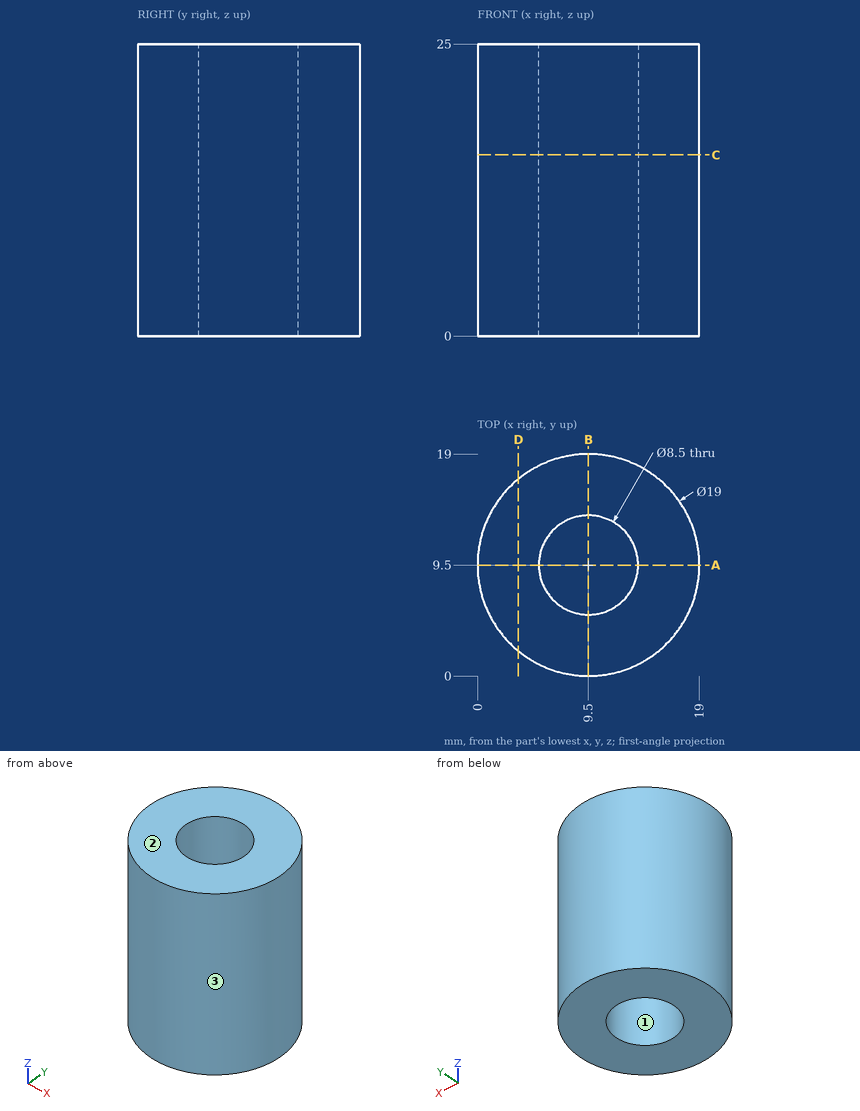
Job drawing, mm, ordinate dimensions from the low corner. One solid piece. Coordinates: 2 decimals unless noted, no trailing zeros. Write each loop counter-clockwise with the first axis right and the second up, starting at its lowest first coordinate (ties: lowest second). Pieces come first, ordered by that corner, then holes. Notation, with made-up numbers: M -17,44.25 L 22,44.25 A4 ccw 22,51.25 Z; hole C 60.25,79 d6. An arc over 180 degrees is marked long. Answer as a JSON object with one key per item and string values. Group by question number.
1) Pin check, flat tips, straight feed: pin 1 Ø1 at (x, z) = (13.5, 14.5) entering from +Y; pin 2 Ø5 at (x, z) = (5, 3) entering from -Y; pin 3 Ø1.5 at (y, z) = (16, 16.5) entering from -X. Stop position of each tip, or through.
2) Wall check: line 1 (Y direction, x = 9.5, z = 17); line 2 (Y direction, x = 7.5, z = 21.25); line 3 (X direction, y = 13, z = 14.75). Give the ranges that are in metal, low to high. Write a range as from..to.
3) Saw through at C-C (z = 15.5). Write the cut outline in (x, y).
4) Saw through at D-D (x = 3.5). Write the cut outline in (y, z).
5) Saw through at A-A (y = 9.5). Write the cut outline in (x, z), plus the area to 4 significant figures.
6) Mould opens along X. For the marked faces 1, 2 and 3 say: +X half, -X half, draft (parallel to the pull), parting line (faces both ways), or undercut.
Values follow:
{
 "1": {"pin 1": "stops at y = 18.33", "pin 2": "stops at y = 0.21", "pin 3": "stops at x = 1.94"},
 "2": {"line 1": "y = 0..5.25, 13.75..19", "line 2": "y = 0.21..5.75, 13.25..18.79", "line 3": "x = 0.67..7.09, 11.91..18.33"},
 "3": {"outline": "C 9.5,9.5 d19; hole C 9.5,9.5 d8.5"},
 "4": {"outline": "M 2.13,0 L 16.87,0 L 16.87,25 L 2.13,25 Z"},
 "5": {"outline": "M 0,0 L 5.25,0 L 5.25,25 L 0,25 Z; M 13.75,0 L 19,0 L 19,25 L 13.75,25 Z", "area": "262.5 mm2"},
 "6": {"face 1": "undercut", "face 2": "draft", "face 3": "parting line"}
}
